from build123d import *

# Parameters (mm, degrees)
SKETCH1_W                    = 14
SKETCH1_H                    = 23
BOSS_EXTRUDE1_DEPTH          = 20
SKETCH2_W                    = 14
SKETCH2_H                    = 10
CUT_EXTRUDE1_DEPTH           = 3
F_3_0_3_DIAMETER_HOLE1_D     = 3
F_3_0_3_DIAMETER_HOLE1_DEPTH = 5
F_3_0_3_DIAMETER_HOLE1_TIP   = 0.901290929
M10X1_0_TAPPED_HOLE1_D       = 9
M10X1_0_TAPPED_HOLE1_DEPTH   = 12
M10X1_0_TAPPED_HOLE1_TIP     = 2.703872786


with BuildPart() as part:
    # Sketch1 → Boss-Extrude1 (new body)
    with BuildSketch(Plane(origin=(0, 0, 0), x_dir=(1, 0, 0), z_dir=(0, 1, 0))):
        with Locations((7, 11.5)):
            Rectangle(SKETCH1_W, SKETCH1_H)
    extrude(amount=-BOSS_EXTRUDE1_DEPTH)

    # Sketch2 → Cut-Extrude1 (cut)
    with BuildSketch(Plane(origin=(0, 0, 0), x_dir=(1, 0, 0), z_dir=(0, 1, 0))):
        with Locations((7, 14)):
            Rectangle(SKETCH2_W, SKETCH2_H)
    extrude(amount=-CUT_EXTRUDE1_DEPTH, mode=Mode.SUBTRACT)

    # Ø3.0 (3) Diameter Hole1
    with Locations(Plane(origin=(0, 0, 0), x_dir=(1, 0, 0), z_dir=(0, 1, 0))):
        with Locations((11, 3), (3, 3)):
            Hole(F_3_0_3_DIAMETER_HOLE1_D / 2, depth=F_3_0_3_DIAMETER_HOLE1_DEPTH)
            with Locations((0, 0, -(F_3_0_3_DIAMETER_HOLE1_DEPTH + F_3_0_3_DIAMETER_HOLE1_TIP / 2))):  # 118° drill point
                Cone(0, F_3_0_3_DIAMETER_HOLE1_D / 2, F_3_0_3_DIAMETER_HOLE1_TIP, mode=Mode.SUBTRACT)

    # M10x1.0 Tapped Hole1
    with Locations(Plane(origin=(0, -20, 0), x_dir=(-1, 0, 0), z_dir=(0, -1, 0))):
        with Locations((-7, 15)):
            Hole(M10X1_0_TAPPED_HOLE1_D / 2, depth=M10X1_0_TAPPED_HOLE1_DEPTH)
            with Locations((0, 0, -(M10X1_0_TAPPED_HOLE1_DEPTH + M10X1_0_TAPPED_HOLE1_TIP / 2))):  # 118° drill point
                Cone(0, M10X1_0_TAPPED_HOLE1_D / 2, M10X1_0_TAPPED_HOLE1_TIP, mode=Mode.SUBTRACT)


solid = part.part
Source: CAD feature listing. Evaluate the final solid. Frame: model axes, mm. A direction names the side the tool comes from. Give positions to 0.01 mm unless a question says otherwise; leave off trailing zeros. Order: outer loops, then holes, each group sorted by start corner. A loop starts at its lowest first (then second) coordinate and runs counter-clockwise, first axis right, second up. Notation, with made-up numbers: (31, 72.25) -> (73, 72.25) arc R10 cw to (73, 91.25) -> close; hole circle Ø9 at (-20.5, 29). An arc over 180 degrees is marked (long way). Write item = value, one per line.
Item 1: Set-up query: faces 1 (the face through (9.419, -13.916, -18.794)), 2 (the face through (0, -10, -11)), 3 (the face through (7, -10, -23)), 4 (the face through (7, -1, -19)), 5 (the face through (12.2, -2.5, -2.1)). Return all of +Z, -Z, +X, -X, +Y, -Y with unobstructed straight access to the full face (end or side cutting, diameter ignored); none if empty.
Check result:
face_1 = -Y
face_2 = +Z, -Z, -X, +Y, -Y
face_3 = -Z, +X, -X, +Y, -Y
face_4 = +X, -X, +Y
face_5 = +Y
Item 2: Ray query, probe 1 along Z at (x, y) = (11, -2.75); probe 2 along Z at (x, y) = (7, -18.75); probe 3 along Z at (x, y) = (11, -3.55). Return the intervals inside material, ascending.
Check result:
probe_1 = -23 to -19, -9 to -4.5, -1.5 to 0
probe_2 = -23 to -19.5, -10.5 to 0
probe_3 = -23 to -4.5, -1.5 to 0
Item 3: Section query A-A (y = -12.75). Output: boundary loops of the cut face in (x, z).
Check result:
outline = (0, -23) -> (14, -23) -> (14, 0) -> (0, 0) -> close; hole circle Ø9 at (7, -15)
Item 4: Section query B-B (y = -4.25). Output: boundary loops of the cut face in (x, z).
Check result:
outline = (0, -23) -> (14, -23) -> (14, 0) -> (0, 0) -> close; hole circle Ø3 at (3, -3); hole circle Ø3 at (11, -3)
Item 5: Mould query, pull axis X, two halves, no side actions, for faces 6 (the face through (2.31, -2.54, -1.67)), 7 (the face through (7, -20, -9)), 8 (the face through (14, -10, -11)). Classes: +X half, -X half, draft (parallel to the pull), parting line (faces both ways), or undercut.
Check result:
face_6 = undercut
face_7 = draft
face_8 = +X half
Item 6: Contact query for flat-ended pins moving along their axis: pin 1 (5.5 mm diameter, centred on x = 7, z = -15, fed in from -Y); pin 2 (2.5 mm diameter, centred on x = 11, z = -3, fed in from +Y). Output: stop coordinate, or through.
Check result:
pin_1 = -6.95
pin_2 = -5.15
